Geometry: final body of the model. Coordinates: model frame, mm. Give positions to 0.01 mm unless a question says otherwise; leave off trailing zeros. Loops run counter-clockwise (first coordinate to the right, second up) from the corner with the lowest first, then second, coordinate; pieces in that order, holes last. Notation, with made-up numbers: (40.25, 39) - (89.25, 39) arc R21 cw to (89.25, 49) - close; hole circle Ø4 at (-16, 15). An arc over 180 degrees is marked (long way). Answer in a Markdown table with one row per item.
from build123d import *

# Parameters (mm, degrees)
F4_DEPTH = 25.4


with BuildPart() as f1:
    # F0 (on Right) → F1 (revolve)
    with BuildSketch(Plane.YZ):
        Polygon((-47.755392, 8.33755), (-47.755392, 0), (65.757208, 0), (65.757208, 6.35), (-43.792992, 6.35), (-43.792992, 8.33755), align=None)
    revolve(axis=Axis((0, -45.774192, 8.33755), (0, -1, 0)))

    # F3 (on offset) → F4 (cut)
    with BuildSketch(Plane.XZ.offset(48.26)):
        with BuildLine():
            ThreePointArc((0, 12.10002), (-3.677915, 8.422106), (0, 4.744191))
            Line((0, 4.744191), (0, 8.422106))
            Line((0, 8.422106), (0, 12.10002))
        make_face()
        with BuildLine():
            Line((0, 8.422106), (0, 4.744191))
            ThreePointArc((0, 4.744191), (2.600678, 5.821427), (3.677915, 8.422106))
            ThreePointArc((3.677915, 8.422106), (2.600678, 11.022784), (0, 12.10002))
            Line((0, 12.10002), (0, 8.422106))
        make_face()
    extrude(amount=-F4_DEPTH, mode=Mode.SUBTRACT)


solid = f1.part
Q1. First-contact query: pin 1 (5 mm diameter, centred on x = 2, y = -27, fed in from -Z); pin 2 (2 mm diameter, centred on x = -6.5, y = -5.5, fed in from +Z). Flat tips, straight axial feed; report the tip coordinate or a pass-through.
Check values:
| item | result |
|---|---|
| pin 1 | z = 0 |
| pin 2 | z = 14.6 |
Q2. Draft query along X for faces 1 (the flat face through (-4, -47.755, 10)), 2 (the cylindrical face through (0.367, 9.795, 16.667)), 3 (the flat face through (2, -22.86, 7)). Return one class per face: pulls with the +X half, pulls with the -X half, needs draft (parallel to the pull), parting line crosses it, or undercut.
Check values:
| item | result |
|---|---|
| face 1 | needs draft |
| face 2 | parting line crosses it |
| face 3 | undercut |
Q3. Cut plane A-A (y = 44). Output: boundary loops of the cut face in (x, z), and give its area (3 significant figures).
Check values:
| item | result |
|---|---|
| outline | circle Ø16.68 at (0, 8.34); hole circle Ø3.98 at (0, 8.34) |
| area | 206 mm² |
Q4. Material intervals for line 1 along X through (y, z) = (24, 8.5); line 2 along X through (y, z) = (44, 6.75); line 3 along Z through (x, y) = (-1.5, 38.5), sorted ascending.
Check values:
| item | result |
|---|---|
| line 1 | -8.34 to -1.98, 1.98 to 8.34 |
| line 2 | -8.19 to -1.2, 1.2 to 8.19 |
| line 3 | 0.14 to 7.03, 9.64 to 16.54 |
Q5. Cut plane B-B (x = 6). Output: boundary loops of the cut face in (y, z), and give its area (3 significant figures).
Check values:
| item | result |
|---|---|
| outline | (-47.76, 2.55) - (65.76, 2.55) - (65.76, 14.13) - (-47.76, 14.13) - close |
| area | 1,310 mm² |
Q6. Cut plane C-C (z = 15.25). Output: boundary loops of the cut face in (x, y), and give its area (3 significant figures).
Check values:
| item | result |
|---|---|
| outline | (-4.66, -47.76) - (4.66, -47.76) - (4.66, 65.76) - (-4.66, 65.76) - close |
| area | 1,060 mm² |
